Build history of the part. All positions in model axes, mm. A direction names the side the tool comes from. Round coordinates to 2 decimals unless told otherwise and drop trailing zeros. Write each loop counter-clockwise with the first axis right and the second up, starting at its lowest first coordinate (ties: lowest second). Pieces come first, ordered by that corner, then holes. Notation, with made-up numbers: (44, 53.5) -> (55, 53.5) arc R14 ccw to (55, 76.5) -> close; hole circle Ø6 at (49, -30). An arc over 180 degrees is marked (long way). Answer in a Markdown table with one row per item.
```python
from build123d import *

# Parameters (mm, degrees)
SKETCH_1_W          = 65
SKETCH_1_H          = 54
SKETCH_1_R          = 1.5
EXTRUDE_1_DEPTH     = 2
SKETCH_2_W          = 65
SKETCH_2_H          = 54
SKETCH_2_W_2        = 61
SKETCH_2_H_2        = 50
EXTRUDE_2_DEPTH     = 50
SKETCH_6_W          = 52
SKETCH_6_H          = 25
SKETCH_6_R          = 1.8
EXTRUDE_3_DEPTH     = 3.5
EXTRUDE_4_DEPTH     = 30
SKETCH_8_R          = 3.1
CUT_EXTRUDE_1_DEPTH = 2.5


with BuildPart() as part:
    # 草图1 → 凸台-拉伸1 (new body)
    with BuildSketch(Plane.XY):
        Rectangle(SKETCH_1_W, SKETCH_1_H)
        with Locations((-26, 18.5)):
            Circle(SKETCH_1_R, mode=Mode.SUBTRACT)
        with Locations(Location((26, 18.5, 0), (0, 0, 180))):
            Circle(SKETCH_1_R, mode=Mode.SUBTRACT)
        with Locations(Location((-26, -18.5, 0), (0, 0, 180))):
            Circle(SKETCH_1_R, mode=Mode.SUBTRACT)
        with Locations((26, -18.5)):
            Circle(SKETCH_1_R, mode=Mode.SUBTRACT)
    extrude(amount=EXTRUDE_1_DEPTH)

    # 草图2 → 凸台-拉伸2 (add)
    with BuildSketch(Plane.XY.offset(2)):
        Rectangle(SKETCH_2_W, SKETCH_2_H)
        Rectangle(SKETCH_2_W_2, SKETCH_2_H_2, mode=Mode.SUBTRACT)
    extrude(amount=EXTRUDE_2_DEPTH)

    # 草图6 → 凸台-拉伸3 (add)
    with BuildSketch(Plane.XY):
        with Locations((0, -39.5)):
            Rectangle(SKETCH_6_W, SKETCH_6_H)
        with Locations((-18.8, -30)):
            Circle(SKETCH_6_R, mode=Mode.SUBTRACT)
        with Locations(Location((18.8, -30, 0), (0, 0, 180))):
            Circle(SKETCH_6_R, mode=Mode.SUBTRACT)
    extrude(amount=EXTRUDE_3_DEPTH)

    # 草图7 → 凸台-拉伸4 (add)
    with BuildSketch(Plane.XY.offset(3.5)):
        Polygon((-24, -27), (-26, -27), (-26, -52), (26, -52), (26, -27), (24, -27), (24, -50), (-24, -50), align=None)
    extrude(amount=EXTRUDE_4_DEPTH)

    # 草图8 → 切除-拉伸1 (cut)
    with BuildSketch(Plane(origin=(0, 0, 0), x_dir=(-1, 0, 0), z_dir=(0, 0, -1))):
        with Locations((-18.8, -30)):
            Circle(SKETCH_8_R)
        with Locations((18.8, -30)):
            Circle(SKETCH_8_R)
    extrude(amount=-CUT_EXTRUDE_1_DEPTH, mode=Mode.SUBTRACT)


solid = part.part
```
Q1. Wall check: line 1 (Y direction, x = -17, z = 16); line 2 (Y direction, x = -18.8, z = 2.9); line 3 (X direction, y = 15, z = 16.5). Give the ranges that are in metal, low to high. Write a range as [from, to].
A:
| item | result |
|---|---|
| line 1 | [-52, -50], [-27, -25], [25, 27] |
| line 2 | [-52, -31.8], [-28.2, -25], [25, 27] |
| line 3 | [-32.5, -30.5], [30.5, 32.5] |
Q2. Saw through at A-A on y = -18.5. Write the cut outline in (x, z), plus the area to 3 significant figures.
A:
| item | result |
|---|---|
| outline | (-32.5, 0) -> (-27.5, 0) -> (-27.5, 2) -> (-30.5, 2) -> (-30.5, 52) -> (-32.5, 52) -> close; (-24.5, 0) -> (24.5, 0) -> (24.5, 2) -> (-24.5, 2) -> close; (27.5, 0) -> (32.5, 0) -> (32.5, 52) -> (30.5, 52) -> (30.5, 2) -> (27.5, 2) -> close |
| area | 318 mm² |
Q3. Saw through at C-C on z = 9.5. Write the cut outline in (x, y).
A:
| item | result |
|---|---|
| outline | (-32.5, -27) -> (-26, -27) -> (-26, -52) -> (26, -52) -> (26, -27) -> (32.5, -27) -> (32.5, 27) -> (-32.5, 27) -> close; hole (-30.5, -25) -> (30.5, -25) -> (30.5, 25) -> (-30.5, 25) -> close; hole (-24, -50) -> (24, -50) -> (24, -27) -> (-24, -27) -> close |
Q4. Saw through at B-B on x = -18.8. Write the cut outline in (y, z).
A:
| item | result |
|---|---|
| outline | (-52, 0) -> (-33.1, 0) -> (-33.1, 2.5) -> (-31.8, 2.5) -> (-31.8, 3.5) -> (-50, 3.5) -> (-50, 33.5) -> (-52, 33.5) -> close; (-28.2, 2.5) -> (-26.9, 2.5) -> (-26.9, 0) -> (27, 0) -> (27, 52) -> (25, 52) -> (25, 2) -> (-25, 2) -> (-25, 52) -> (-27, 52) -> (-27, 3.5) -> (-28.2, 3.5) -> close |
Q5. Saw through at D-D on x = 3.5. Write the cut outline in (y, z), plus the area to 4 significant figures.
A:
| item | result |
|---|---|
| outline | (-52, 0) -> (27, 0) -> (27, 52) -> (25, 52) -> (25, 2) -> (-25, 2) -> (-25, 52) -> (-27, 52) -> (-27, 3.5) -> (-50, 3.5) -> (-50, 33.5) -> (-52, 33.5) -> close |
| area | 455.5 mm² |
Q6. Two-plate mould, pull along Y, no slides. Class faces 1 (the flat face through (-3, -26, 52)), 2 (the flat face through (17, -31, 2.5)), 3 (the flat face through (0, -52, 17)), 4 (the flat face through (0, 27, 26)): released by +Y, released by -Y, zero draft, split by the parting line, or undercut.
A:
| item | result |
|---|---|
| face 1 | zero draft |
| face 2 | undercut |
| face 3 | released by -Y |
| face 4 | released by +Y |
Q7. Which spindle directions (+Z, -Z, +X, -X, +Y, -Y) get a long thin tool onto all of the face, cutting with end or side? Do faces 5 (the cylindrical face through (21.08, -27.9, 1.23)), 6 (the flat face through (0, -51, 33.5)), 7 (the flat face through (0, -25, 27)). Say none if no direction does.
A:
| item | result |
|---|---|
| face 5 | -Z |
| face 6 | +Z, +X, -X, -Y |
| face 7 | +Z |
Q8. Drop flat-ended pins along their axis: P1, Ø5, axis at x = -26, y = -18.5, coming from the -Z side; P2, Ø4, axis at x = -26, y = 18.5, coming from the +Z side; P3, Ø11.5, axis at x = -9.5, y = -34, coming from the +Z side; P4, Ø3, axis at x = 20, y = -29, coming from the -Z side. Give the stop position or say it passes through.
A:
| item | result |
|---|---|
| P1 | z = 0 |
| P2 | z = 2 |
| P3 | z = 3.5 |
| P4 | z = 2.5 |
